Part model, mm, in its own coordinate system. A direction names the side the tool comes from. Coordinates: 2 decimals unless noted, no trailing zeros. Loops run counter-clockwise (first coordinate to the right, second up) from the corner with the lowest first, then second, coordinate; pieces in that order, holes last. Notation, with made-up numbers: (61, 37.25) - (92, 37.25) arc R10 cw to (92, 55.25) - close; hole circle Ø11 at (60, 7). An arc over 180 degrees is marked (long way). Use a Markdown table: item, result. Add a question column.
1) Tool access for faces 4 (the face through (2.528, -6.45, -21.204)), 5 (the face through (1.846, 3.549, -18.14)), 6 (the face through (-6.454, 2.528, -21.204)): list every direction of +Z, -Z, +X, -X, +Y, -Y with a clear straight run to the whole face (end or side of a thin tool).
2) Drop flat-ended pins along their axis: P1, Ø2.5, axis at x = -1, y = -1, coming from the -Z side; P2, Ø10, axis at x = -6, z = -3.5, coming from the -Y side; P3, Ø4, axis at x = -3, z = -8, coming from the +Y side. Give the stop position or say it passes through.
3) Probe probe 1 along Z at (x, y) = (0, -4.75); probe 2 along Z at (x, y) = (-2, -3.75); probe 3 along Y at (x, z) = (0, -17). List the from-to ranges inside material, lowest first. Write a range as [from, to].
4) Band-saw the part on A-A (y = 0). Give the cut face in (x, z), plus the area to 3 significant figures.
5) Band-saw the part on C-C (z = -24). Give the cut face in (x, y).
6) Pull direction Z, two halves, no side cores. Call faces 1 (the face through (-6.45, 2.45, -14.01)), 2 (the face through (0, 0, 4)), 3 (the face through (0, 0, -8)): +Z half, -Z half, draft (parallel to the pull), parting line (faces both ways), or undercut.
7) Band-saw the part on D-D (z = -9). Give the cut face in (x, y), plus the area to 3 significant figures.
from build123d import *

# Parameters (mm, degrees)
SKETCH051_R       = 10
PAD041_DEPTH      = 4
PAD041_DEPTH_BACK = 28
SKETCH052_R       = 4
POCKET_DEPTH      = 20
SKETCH053_R       = 2.65
POCKET005_DEPTH   = 27
SKETCH054_R       = 2.65
POCKET006_DEPTH   = 11


with BuildPart() as part:
    # Sketch051 → Pad041 (new body, two sides)
    with BuildSketch(Plane.XY) as pad041_sk:
        Circle(SKETCH051_R)
    extrude(amount=PAD041_DEPTH)
    extrude(pad041_sk.sketch, amount=-PAD041_DEPTH_BACK)

    # Sketch052 (on Face2 of Pad041) → Pocket (cut)
    with BuildSketch(Plane(origin=(0, 0, -28), x_dir=(1, 0, 0), z_dir=(0, 0, -1))):
        Circle(SKETCH052_R)
    extrude(amount=-POCKET_DEPTH, mode=Mode.SUBTRACT)

    # Sketch053 → Pocket005 (cut)
    with BuildSketch(Plane.XZ):
        with Locations((0, -22)):
            Circle(SKETCH053_R)
        with Locations((0, -13)):
            Circle(SKETCH053_R)
    extrude(amount=POCKET005_DEPTH, mode=Mode.SUBTRACT)

    # Sketch054 → Pocket006 (cut)
    with BuildSketch(Plane.YZ):
        with Locations((0, -13)):
            Circle(SKETCH054_R)
        with Locations((0, -22)):
            Circle(SKETCH054_R)
    extrude(amount=-POCKET006_DEPTH, mode=Mode.SUBTRACT)


solid = part.part
Answer block:
| question | item | result |
|---|---|---|
| 1 | face 4 | -Y |
| 1 | face 5 | -Z |
| 1 | face 6 | -X |
| 2 | P1 | z = -8 |
| 2 | P2 | y = -9.95 |
| 2 | P3 | y = 9.95 |
| 3 | probe 1 | [-28, -24.65], [-19.35, -15.65], [-10.35, 4] |
| 3 | probe 2 | [-28, -23.74], [-20.26, -14.74], [-11.26, 4] |
| 3 | probe 3 | [-10, -4], [4, 10] |
| 4 | outline | (-10, -28) - (-4, -28) - (-4, -24.65) - (-10, -24.65) - close; (-10, -19.35) - (-4, -19.35) - (-4, -15.65) - (-10, -15.65) - close; (-10, -10.35) - (-4, -10.35) - (-4, -8) - (4, -8) - (4, -28) - (10, -28) - (10, 4) - (-10, 4) - close |
| 4 | area | 416 mm2 |
| 5 | outline | (-9.85, -1.74) arc R10 ccw to (-1.74, -9.85) - (-1.74, -3.6) arc R4 cw to (-3.6, -1.74) - close; (-9.85, 1.74) - (-3.6, 1.74) arc R4 cw (long way) to (1.74, -3.6) - (1.74, -9.85) arc R10 ccw (long way) to start |
| 6 | face 1 | undercut |
| 6 | face 2 | +Z half |
| 6 | face 3 | -Z half |
| 7 | outline | circle Ø20 at (0, 0); hole circle Ø8 at (0, 0) |
| 7 | area | 264 mm2 |
